Read the model definition and answer for the solid it produces. Units are mm, in the model's axes. A direction names the side the tool comes from. Give positions to 0.01 mm unless a question says otherwise; leave off trailing zeros. Order: outer loops, then holes, each group sorted by start corner. A loop starts at its lowest first (then second) coordinate and runs counter-clockwise, first axis right, second up. Notation, with made-up numbers: (-36, -37.75) - (6, -37.75) arc R20 cw to (6, -33.75) - close; hole circle Ø7 at (1, 63.25). An arc over 180 degrees is marked (long way). Write item = value, one per line.
```python
from build123d import *

# Parameters (mm, degrees)
F1_W = 7.25
F1_H = 1
F4_D = 4.4
F5_D = 4.4
F6_D = 4.4
F7_D = 4.4


with BuildPart() as f2:
    # F1 (on Front) → F2 (revolve)
    with BuildSketch(Plane.XZ):
        Polygon((11.5, 1), (11.5, 0), (23.75, 0), (23.75, 1), (16.5, 1), align=None)
        with Locations((20.125, 1.5)):
            Rectangle(F1_W, F1_H)
    revolve(axis=Axis((0, 0, 1.627581194), (0, 0, -1)))

    # F4 (through all)
    with Locations(Plane(origin=(0, 0, 0), x_dir=(1, 0, 0), z_dir=(0, 0, -1))):
        with Locations((19.5, 0)):
            Hole(F4_D / 2)

    # F5 (through all)
    with Locations(Plane(origin=(0, 0, 0), x_dir=(1, 0, 0), z_dir=(0, 0, -1))):
        with Locations((0, 19.5)):
            Hole(F5_D / 2)

    # F6 (through all)
    with Locations(Plane(origin=(0, 0, 0), x_dir=(1, 0, 0), z_dir=(0, 0, -1))):
        with Locations((-19.5, 0)):
            Hole(F6_D / 2)

    # F7 (through all)
    with Locations(Plane(origin=(0, 0, 0), x_dir=(1, 0, 0), z_dir=(0, 0, -1))):
        with Locations((0, -19.5)):
            Hole(F7_D / 2)


solid = f2.part
```
1. Flat-ended cylindrical pins translate along their axes: pin 1 (4 mm diameter, centred on x = 0, y = 19.5, fed in from +Z); pin 2 (3 mm diameter, centred on x = -6, y = 11, fed in from +Z). Find the tip coordinate at first contact, or state that the pin passes through.
Recorded:
pin_1 = through
pin_2 = 1
2. Determine the mould class of faces 1 (the face through (5, -16, 2)), 2 (the face through (-1.5, -11.4, 0.5)), 3 (the face through (-5.149, 23.185, 1.014)) for opening direction X: +X half, -X half, draft (parallel to the pull), parting line (faces both ways), or undercut.
Recorded:
face_1 = draft
face_2 = undercut
face_3 = parting line
3. Section D-D (x = 5) is taken. Determine the outline of the cut face in (y, z), and give its area (3 significant figures).
Recorded:
outline = (-23.22, 0) - (-10.36, 0) - (-10.36, 1) - (-15.72, 1) - (-15.72, 2) - (-23.22, 2) - close; (10.36, 0) - (23.22, 0) - (23.22, 2) - (15.72, 2) - (15.72, 1) - (10.36, 1) - close
area = 40.7 mm^2
4. Section B-B (y = -19.5) is taken. Determine the outline of the cut face in (x, z).
Recorded:
outline = (-13.56, 0) - (-2.2, 0) - (-2.2, 2) - (-13.56, 2) - close; (2.2, 0) - (13.56, 0) - (13.56, 2) - (2.2, 2) - close
5. Straight lines are drawn through the part: L1, parallel to Y at x = 0, z = 0.5; L2, parallel to Y at x = 0, z = 1.7; L3, parallel to Y at x = -4, z = 0.5. For each, find the intervals that lie inside material, in ascending order. Write a range as [from, to].
Recorded:
L1 = [-23.75, -21.7], [-17.3, -11.5], [11.5, 17.3], [21.7, 23.75]
L2 = [-23.75, -21.7], [-17.3, -16.5], [16.5, 17.3], [21.7, 23.75]
L3 = [-23.41, -10.78], [10.78, 23.41]
6. Section A-A (x = 0) is taken. Determine the outline of the cut face in (y, z).
Recorded:
outline = (-23.75, 0) - (-21.7, 0) - (-21.7, 2) - (-23.75, 2) - close; (-17.3, 0) - (-11.5, 0) - (-11.5, 1) - (-16.5, 1) - (-16.5, 2) - (-17.3, 2) - close; (11.5, 0) - (17.3, 0) - (17.3, 2) - (16.5, 2) - (16.5, 1) - (11.5, 1) - close; (21.7, 0) - (23.75, 0) - (23.75, 2) - (21.7, 2) - close
7. Section C-C (z = 0.3) is taken. Determine the outline of the cut face in (x, y), and give its area (3 significant figures).
Recorded:
outline = circle Ø47.5 at (0, 0); hole circle Ø4.4 at (-19.5, 0); hole circle Ø23 at (0, 0); hole circle Ø4.4 at (0, -19.5); hole circle Ø4.4 at (0, 19.5); hole circle Ø4.4 at (19.5, 0)
area = 1,300 mm^2
8. For faces 4 (the face through (0.477, -17.352, 1.014)), 5 (the face through (15.24, 6.32, 1.51)), determine the directions among +Z, -Z, +X, -X, +Y, -Y from which every point of the face is accessible in a straight line to the end or side of a thin tool.
Recorded:
face_4 = +Z, -Z
face_5 = +Z
